Could you check a few things on this model? Use its own coordinates, in mm. A direction names the side the tool comes from. Round coordinates to 2 decimals unless told otherwise and drop trailing zeros. Loops run counter-clockwise (first coordinate to the right, second up) from the corner with the lowest first, then second, coordinate; pieces in that order, holes last. Notation, with made-up numbers: M -1,67.5 L 45,67.5 A32 ccw 45,97.5 Z; hole C 75.25,89.25 d2. An arc over 180 degrees is marked long. One line per item, written item: value. Start each with the question number.
Q1. Thinking about a two-plate mould opening in X: for faces 3 (the face through (-22, 3, 71.91)), 4 (the face through (66.364, 3.131, 39.034)), 5 (the face through (-51.38, 3.22, -54.83)), 6 (the face through (-66.364, 3.131, -39.034)), which applies, released by +X, released by -X, zero draft, split by the parting line, or undercut?
Q2. I'm going to push flat-ended pins straight in: pin 1 Ø1.6 at (y, z) = (4, 73.5) entering from +X; pin 2 Ø1.5 at (y, z) = (1, 16.5) entering from +X; pin 3 Ø1.6 at (y, z) = (2.5, -74) entering from +X. Where does each tip first touch, or does it pass through?
Q3. Which directions (+Z, -Z, +X, -X, +Y, -Y) give clear straight access to the entire face, cutting with the end or side of a thin tool? Please do faces 1 (the face through (1, 3, -76.99)), 2 (the face through (-51.38, 3.22, 54.83)).
Q4. Please list where these lines run through material, in increasing order: line 1 along Z through (x, y) = (-20, 2); line 2 along X through (y, z) = (3.25, -50); line 3 along X through (y, z) = (4.5, 62.5).
Q5. Imagine slicing it at C-C (y = 3.75). Give the number of separate pieces and of enclosed holes in the cut face, then the cut area to 3 significant figures.
Q6. Imagine slicing it at D-D (z = -35.5). Please give me the cut outline in (x, y), then the cut area to 3 significant figures.
Q7. Imagine slicing it at A-A (x = -11.5). Please give me the cut outline in (y, z).
Q8. Imagine slicing it at B-B (z = -11.5). Please give me the cut outline in (x, y).
from build123d import *

# Parameters (mm, degrees)
BOSS_EXTRUDE1_DEPTH = 6.35
SKETCH2_W           = 24.892
SKETCH2_H           = 3.175
CUT_EXTRUDE1_DEPTH  = 7.35


with BuildPart() as part:
    # Sketch1 → Boss-Extrude1 (new body)
    with BuildSketch(Plane(origin=(0, 0, 0), x_dir=(1, 0, 0), z_dir=(0, 1, 0))):
        Polygon((-88.9, 0), (-44.45, -76.989658396), (44.45, -76.989658396), (88.9, 0), (44.45, 76.989658396), (-44.45, 76.989658396), align=None)
    extrude(amount=BOSS_EXTRUDE1_DEPTH)

    # Sketch2 → Cut-Extrude1 (cut, through all)
    with BuildSketch(Plane(origin=(0, 6.35, 0), x_dir=(1, 0, 0), z_dir=(0, 1, 0))):
        Polygon((-79.484090949, -6.148832876), (-82.233721606, -7.736332876), (-69.787721606, -29.293437227), (-67.038090949, -27.705937227), align=None)
        Polygon((-45.067090949, -65.76082552), (-47.816721606, -67.34832552), (-60.262721606, -45.791221169), (-57.513090949, -44.203721169), align=None)
        Polygon((-45.067090949, 65.76082552), (-47.816721606, 67.34832552), (-60.262721606, 45.791221169), (-57.513090949, 44.203721169), align=None)
        Polygon((-69.787721606, 29.293437227), (-67.038090949, 27.705937227), (-79.484090949, 6.148832876), (-82.233721606, 7.736332876), align=None)
        with Locations((21.971, 73.497158396)):
            Rectangle(SKETCH2_W, SKETCH2_H)
        with Locations((-21.971, 73.497158396)):
            Rectangle(SKETCH2_W, SKETCH2_H)
        Polygon((79.484090949, 6.148832876), (82.233721606, 7.736332876), (69.787721606, 29.293437227), (67.038090949, 27.705937227), align=None)
        Polygon((60.262721606, 45.791221169), (57.513090949, 44.203721169), (45.067090949, 65.76082552), (47.816721606, 67.34832552), align=None)
        Polygon((45.067090949, -65.76082552), (47.816721606, -67.34832552), (60.262721606, -45.791221169), (57.513090949, -44.203721169), align=None)
        Polygon((69.787721606, -29.293437227), (67.038090949, -27.705937227), (79.484090949, -6.148832876), (82.233721606, -7.736332876), align=None)
        with Locations((-21.971, -73.497158396)):
            Rectangle(SKETCH2_W, SKETCH2_H)
        with Locations((21.971, -73.497158396)):
            Rectangle(SKETCH2_W, SKETCH2_H)
    extrude(amount=-CUT_EXTRUDE1_DEPTH, mode=Mode.SUBTRACT)


solid = part.part
Report:
1. face 3: undercut
1. face 4: released by +X
1. face 5: undercut
1. face 6: released by -X
2. pin 1: stops at x = 46.93
2. pin 2: stops at x = 79.81
2. pin 3: stops at x = 46.64
3. face 1: -Z, +X, -X, +Y, -Y
3. face 2: +Y, -Y
4. line 1: z = -76.99 to -75.08, -71.91 to 71.91, 75.08 to 76.99
4. line 2: x = -60.03 to -57.83, -54.17 to 54.17, 57.83 to 60.03
4. line 3: x = -52.82 to -50.62, -46.95 to 46.95, 50.62 to 52.82
5. separate pieces: 1
5. enclosed holes: 12
5. area: 19,600 mm²
6. outline: M -68.4,0 L 68.4,0 L 68.4,6.35 L -68.4,6.35 Z
6. area: 869 mm²
7. outline: M 0,-76.99 L 6.35,-76.99 L 6.35,-75.08 L 0,-75.08 Z; M 0,-71.91 L 6.35,-71.91 L 6.35,71.91 L 0,71.91 Z; M 0,75.08 L 6.35,75.08 L 6.35,76.99 L 0,76.99 Z
8. outline: M -82.26,0 L -80.06,0 L -80.06,6.35 L -82.26,6.35 Z; M -76.39,0 L 76.39,0 L 76.39,6.35 L -76.39,6.35 Z; M 80.06,0 L 82.26,0 L 82.26,6.35 L 80.06,6.35 Z
